```python
from build123d import *

# Parameters (mm, degrees)
F0_R     = 3.25
F1_DEPTH = 2.9


# Not quite as in the source:
# - ends of sketch curves that miss each other by under 0.0002 mm in the source are joined


with BuildPart() as f1:
    # F0 (on Top) → F1 (new body)
    with BuildSketch(Plane.XY):
        with BuildLine():
            ThreePointArc((-44.7213694768, -87.2696897378), (-35.3282259069, -78.6355727138), (-22.6261189451, -77.437406766))
            ThreePointArc((-22.6261189451, -77.437406766), (-3.9584138319, -79.9784717794), (14.8526419701, -78.9371528028))
            ThreePointArc((14.8526419701, -78.9371528028), (27.4184013914, -81.1464387638), (36.0916099164, -90.5034990376))
            Line((36.0916099164, -90.5034990376), (43.056946, -105.982018))
            ThreePointArc((43.056946, -105.982018), (56.6433108611, -112.762891287), (65.9972675289, -100.8015700101))
            ThreePointArc((65.9972675289, -100.8015700101), (70.3098677706, -65.4781038722), (84.4013998186, -32.8012868888))
            ThreePointArc((84.4013998186, -32.8012868888), (98.9543772418, 21.9475596078), (81.1058809507, 75.7123879655))
            ThreePointArc((81.1058809507, 75.7123879655), (78.4915241697, 80.9342205742), (77.4969704068, 86.68861601))
            ThreePointArc((77.4969704068, 86.68861601), (74.5710678119, 93.5134278119), (67.7462419947, 96.4393277843))
            ThreePointArc((67.7462419947, 96.4393277843), (61.9918305742, 97.4338841697), (56.7700159448, 100.0482399211))
            ThreePointArc((56.7700159448, 100.0482399211), (51.7741884012, 103.3250206324), (46.589782882, 106.2944757787))
            ThreePointArc((46.589782882, 106.2944757787), (39.1449717302, 113.1782098516), (36.0328533434, 122.8283870191))
            Line((36.0328533434, 122.8283870191), (34.976746, 141.777077))
            ThreePointArc((34.976746, 141.777077), (22.4266252093, 155.7447750088), (6.0736789634, 146.5152930146))
            Line((6.0736789634, 146.5152930146), (-0.977233, 128.895637))
            ThreePointArc((-0.977233, 128.895637), (-7.0076373704, 120.7442287718), (-16.2606700755, 116.5978324535))
            ThreePointArc((-16.2606700755, 116.5978324535), (-37.4411993299, 110.5892726198), (-56.7700327307, 100.0482376153))
            ThreePointArc((-56.7700327307, 100.0482376153), (-61.9918290994, 97.4338843258), (-67.7462240106, 96.4393304314))
            ThreePointArc((-67.7462240106, 96.4393304314), (-74.5710678119, 93.5134278119), (-77.4969677843, 86.6886019947))
            ThreePointArc((-77.4969677843, 86.6886019947), (-78.4915233258, 80.9342200994), (-81.1058789211, 75.7124059448))
            ThreePointArc((-81.1058789211, 75.7124059448), (-98.9973221942, 19.6705072268), (-81.9321709394, -36.6284899589))
            ThreePointArc((-81.9321709394, -36.6284899589), (-72.1246020826, -62.3015797591), (-74.7927308672, -89.6544180452))
            Line((-74.7927308672, -89.6544180452), (-77.359069, -97.188309))
            ThreePointArc((-77.359069, -97.188309), (-70.8446126339, -112.0362432093), (-55.4854090748, -106.8406649589))
            Line((-55.4854090748, -106.8406649589), (-44.7213694768, -87.2696897378))
        make_face()
        with Locations((-66, -101.05764)):
            Circle(F0_R, mode=Mode.SUBTRACT)
        with BuildLine():
            ThreePointArc((-52.5642634566, -89.0792787489), (-55.6931843813, -91.5103563164), (-59.6084751577, -90.9014372506))
            ThreePointArc((-59.6084751577, -90.9014372506), (-61.3402321592, -89.9993144635), (-63.1953610952, -89.3899923959))
            ThreePointArc((-63.1953610952, -89.3899923959), (-66.2453647932, -87.2123878479), (-66.9254446607, -83.5270150694))
            ThreePointArc((-66.9254446607, -83.5270150694), (-65.7348712362, -74.7077507104), (-65.7415821416, -65.8084890097))
            ThreePointArc((-65.7415821416, -65.8084890097), (-63.1835418456, -61.0980378443), (-57.8323762514, -61.4094713493))
            ThreePointArc((-57.8323762514, -61.4094713493), (-52.4648777131, -65.01260773), (-46.8736571173, -68.2577562181))
            ThreePointArc((-46.8736571173, -68.2577562181), (-44.4460535436, -71.2446768384), (-44.8599474566, -75.0713907489))
            Line((-44.8599474566, -75.0713907489), (-52.5642634566, -89.0792787489))
        make_face(mode=Mode.SUBTRACT)
        with Locations((-67.5, -48.55764)):
            Circle(F0_R, mode=Mode.SUBTRACT)
        with Locations((54, -101.05764)):
            Circle(F0_R, mode=Mode.SUBTRACT)
        with BuildLine():
            ThreePointArc((55.7668649484, -62.8565289244), (61.4137793469, -62.8660371217), (63.450485388, -68.1328730913))
            ThreePointArc((63.450485388, -68.1328730913), (61.7927741104, -76.349981087), (60.66398801, -84.656313001))
            ThreePointArc((60.66398801, -84.656313001), (58.8502515766, -88.0169614514), (55.1933120197, -89.1171158029))
            ThreePointArc((55.1933120197, -89.1171158029), (51.7212938161, -89.2759806038), (48.4404431818, -90.4231993478))
            ThreePointArc((48.4404431818, -90.4231993478), (44.4890186454, -90.7173209458), (41.5643552496, -88.0440028877))
            Line((41.5643552496, -88.0440028877), (37.204438, -78.355278))
            ThreePointArc((37.204438, -78.355278), (37.0976309763, -74.5077318057), (39.7561530447, -71.7243331019))
            ThreePointArc((39.7561530447, -71.7243331019), (47.9668749837, -67.6612132767), (55.7668649484, -62.8565289244))
        make_face(mode=Mode.SUBTRACT)
        with Locations((67.5, -48.55764)):
            Circle(F0_R, mode=Mode.SUBTRACT)
        with BuildLine():
            ThreePointArc((-57.9428097278, 83.4995499162), (-57.3338219129, 84.7875612773), (-56.3862887981, 85.8515257605))
            ThreePointArc((-56.3862887981, 85.8515257605), (-1.4091e-06, 106.44236), (56.3862897755, 85.8515247336))
            ThreePointArc((56.3862897755, 85.8515247336), (57.3338226492, 84.7875616758), (57.9428104466, 83.4995508296))
            ThreePointArc((57.9428104466, 83.4995508296), (60.4289318502, 79.371292526), (64.557188973, 76.8851709122))
            ThreePointArc((64.557188973, 76.8851709122), (65.8452017985, 76.276181568), (66.9091657605, 75.3286487981))
            ThreePointArc((66.9091657605, 75.3286487981), (87.5, 18.94236), (66.9091656417, -37.443928698))
            ThreePointArc((66.9091656417, -37.443928698), (65.8452017985, -38.391461568), (64.5571911108, -39.00044936))
            ThreePointArc((64.5571911108, -39.00044936), (60.4289318502, -41.486572526), (57.942810631, -45.6148298864))
            ThreePointArc((57.942810631, -45.6148298864), (57.3338226492, -46.9028416758), (56.3862897981, -47.9668057605))
            ThreePointArc((56.3862897981, -47.9668057605), (-1.4091e-06, -68.55764), (-56.3862919305, -47.9668029175))
            ThreePointArc((-56.3862919305, -47.9668029175), (-57.3338219129, -46.9028412773), (-57.9428097278, -45.6148299162))
            ThreePointArc((-57.9428097278, -45.6148299162), (-60.4289318502, -41.486572526), (-64.5571880596, -39.0004511935))
            ThreePointArc((-64.5571880596, -39.0004511935), (-65.8452006758, -38.3914616492), (-66.9091647605, -37.4439287981))
            ThreePointArc((-66.9091647605, -37.4439287981), (-87.5, 18.94236), (-66.9091638256, 75.328650853))
            ThreePointArc((-66.9091638256, 75.328650853), (-65.8452006758, 76.2761816492), (-64.5571898296, 76.8851694466))
            ThreePointArc((-64.5571898296, 76.8851694466), (-60.4289318502, 79.371292526), (-57.9428097278, 83.4995499162))
        make_face(mode=Mode.SUBTRACT)
        with Locations((-67.5, 86.44236)):
            Circle(F0_R, mode=Mode.SUBTRACT)
        with BuildLine():
            ThreePointArc((10.7869112155, 143.4660389647), (21.6986369647, 151.3040387845), (29.5366367845, 140.3923130353))
            Line((29.5366367845, 140.3923130353), (29.213074, 138.418678))
            ThreePointArc((29.213074, 138.418678), (18.3013640353, 130.5806802155), (10.4633642155, 141.4924059647))
            Line((10.4633642155, 141.4924059647), (10.7869112155, 143.4660389647))
        make_face(mode=Mode.SUBTRACT)
        with Locations((67.5, 86.44236)):
            Circle(F0_R, mode=Mode.SUBTRACT)
    extrude(amount=F1_DEPTH)


solid = f1.part
```
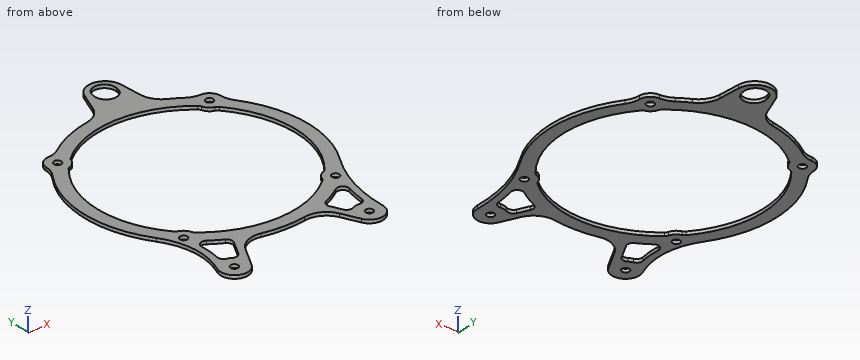
Build history of the part. All positions in model axes, mm. Round coordinates to 2 decimals unless told otherwise and drop trailing zeros.
Item 1: Saw through at A-A (z = 1.1). State how many separate pieces and enclosed holes the cut face has, then the cut area to 3 significant figures.
Item 2: Drill centre lines: line 1 along Y through (x, z) = (-67.5, 2.25); line 2 along X through (y, z) = (-99, 1.2); line 3 along X through (y, z) = (-75, 1.2). Where is each one in solid material? Low to high.
Item 3: Pin check, flat tip, straight feed: P1, Ø6, axis at x = 54, y = -101.06, coming from the +Z side. Stop position of the tip, or through.
Worked answers:
1. separate pieces: 1
1. enclosed holes: 10
1. area: 9,830 mm2
2. line 1: y = -112.96 to -103.94, -98.17 to -51.81, -45.31 to -36.74, 74.62 to 83.19, 89.69 to 96.45
2. line 2: x = -77.82 to -68.52, -63.48 to -51.17, 39.92 to 51.48, 56.52 to 65.97
2. line 3: x = -71.77 to -65.76, -44.82 to 36.94, 62.03 to 68.13
3. P1: passes through
